Input: part model. Units: mm. Frame: model coordinates. Give positions to 0.01 mm unless a question says otherwise; leave off trailing zeros. Loops run counter-clockwise (first coordinate to the right, second up) from the corner with the lowest first, then second, coordinate; pieces in that order, holes last. Notation, with made-up numbers: (86.25, 77) - (110.25, 77) arc R23 ccw to (110.25, 92) - close; hole circle Ø2 at (-6, 61). An arc over 180 degrees is marked (long way). Answer as a JSON object with one key per item and string values. Group by question number.
(1) Section query B-B (x = -3). Return loops of the section in (y, z), plus the area to 3 significant figures.
(2) Section query A-A (z = 45.5). Return loops of the section in (x, y).
(3) Section query C-C (y = 2.3). Count the separate pieces of the cut face and the enclosed holes in it, plus the area to 3 significant figures.
(4) Material intervals for L1, parallel to X at y = 4.15, z = -12.5; L2, parallel to X at y = 4.6, z = -43; L3, parallel to X at y = 1.4, z = 3, sorted ascending.
Autodesk Inventor part; units mm, degrees
ref_plane "YZ Plane" through (0, 0, 0) normal (1, 0, 0) x (0, 1, 0)
ref_plane "XZ Plane" through (0, 0, 0) normal (0, 1, 0) x (-1, 0, 0)
ref_plane "XY Plane" through (0, 0, 0) normal (0, 0, 1) x (1, 0, 0)
sketch "Sketch1" plane through (0, 0, 0) normal (0, 1, 0) x (-1, 0, 0)
  line L0 (-50.8, 63.5) -> (50.8, 63.5)
  line L1 (50.8, 63.5) -> (50.8, -63.5)
  line L2 (50.8, -63.5) -> (-50.8, -63.5)
  line L3 (-50.8, -63.5) -> (-50.8, 63.5)
  line L4 (-50.8, 63.5) -> (50.8, -63.5) construction
  line L5 (50.8, 63.5) -> (-50.8, -63.5) construction
  point P0 (0, 0)
  point P1 (0, 0)
  dimension "d0" = 101.6
  dimension "d1" = 127
extrude "Plate1" add sketch "Sketch1" along normal blind 5.08
sketch "Sketch2" plane through (0, 5.08, 0) normal (0, 1, 0) x (1, 0, 0)
  line L0 (-50.8, 63.5) -> (50.8, 63.5) construction
  line L1 (0, 63.5) -> (0, -63.5) construction
  line L2 (50.8, -63.5) -> (-50.8, -63.5) construction
  line L3 (-50.8, -63.5) -> (-50.8, 63.5) construction
  point P0 (0, 0)
  point P1 (-37.338, -38.1)
  point P2 (-37.338, -18.542)
  point P3 (37.338, -38.1)
  point P4 (37.338, -18.542)
  dimension "d5" = 19.558
  dimension "d6" = 13.462
  dimension "d18" = 25.4
hole "MotorScrews" at (-37.338, 5.08, 38.1) at (-37.338, 5.08, 18.542) at (37.338, 5.08, 38.1) at (37.338, 5.08, 18.542) direction (0, -1, 0) diameter 3.2766 end through all
sketch "Sketch3" plane through (0, 5.08, 0) normal (0, 1, 0) x (1, 0, 0)
  line L0 (-18.5, -59.9042) -> (18.5, -59.9042)
  line L1 (18.5, -59.9042) -> (18.5, 21.0958)
  line L2 (18.5, 21.0958) -> (-18.5, 21.0958)
  line L3 (-18.5, 21.0958) -> (-18.5, -59.9042)
  line L4 (-18.5, -59.9042) -> (18.5, 21.0958) construction
  line L5 (18.5, -59.9042) -> (-18.5, 21.0958) construction
  point P0 (0, 0)
  point P1 (0, -19.4042)
  point P2 (0, -19.4042)
  dimension "d14" = 37
  dimension "d15" = 81
extrude "BatteryHole" cut sketch "Sketch3" against normal blind 5.08
sketch "Sketch4" plane through (0, 5.08, 0) normal (0, 1, 0) x (1, 0, 0)
  line L0 (18.5, -59.9042) -> (-18.5, -59.9042)
  line L1 (-25.0073, -30.5582) -> (25.0073, -30.5582)
  line L2 (25.0073, -30.5582) -> (25.0073, -24.8469)
  line L3 (25.0073, -24.8469) -> (-25.0073, -24.8469)
  line L4 (-25.0073, -24.8469) -> (-25.0073, -30.5582)
  line L5 (-25.0073, -30.5582) -> (25.0073, -24.8469) construction
  line L6 (25.0073, -30.5582) -> (-25.0073, -24.8469) construction
  point P0 (0, 0)
  point P1 (0, -27.7026)
  point P2 (0, -27.7026)
extrude "MotorWireHoles" cut sketch "Sketch4" against normal blind 5.08
sketch "Sketch5" plane through (0, 5.08, 0) normal (0, 1, 0) x (1, 0, 0)
  line L0 (0, 0) -> (0, 25.4) construction
  line L1 (-50.8, 63.5) -> (50.8, 63.5)
  point P0 (-24.4983, 2.3368)
  point P1 (24.4983, 2.3368)
  point P2 (-24.4983, 60.325)
  point P3 (24.4983, 60.325)
  dimension "d21" = 25.4
  dimension "d22" = 48.9966
  dimension "d23" = 57.9882
  dimension "d24" = 3.175
hole "PiScrews" at (-24.4983, 5.08, -2.3368) at (24.4983, 5.08, -2.3368) at (-24.4983, 5.08, -60.325) at (24.4983, 5.08, -60.325) direction (0, -1, 0) diameter 2.8956 end through all
sketch "Sketch6" plane through (0, 5.08, 0) normal (0, 1, 0) x (1, 0, 0)
  line L0 (-15.4305, 17.2899) -> (-15.4305, 42.6899) construction
  line L1 (-26.2255, 57.1039) -> (-23.0505, 57.1039)
  line L2 (-23.0505, 57.1039) -> (-23.0505, 6.3039)
  line L3 (-23.0505, 6.3039) -> (-26.2255, 6.3039)
  line L4 (-26.2255, 6.3039) -> (-26.2255, 57.1039)
  circle A0 centre (-24.4983, 60.325) radius 1.4478
  line L5 (-4.6355, 57.1039) -> (-7.8105, 57.1039)
  line L6 (-7.8105, 57.1039) -> (-7.8105, 23.8538)
  line L7 (-7.8105, 23.8538) -> (-4.6355, 23.8538)
  line L8 (-4.6355, 23.8538) -> (-4.6355, 57.1039)
  dimension "d33" = 3.175
  dimension "d34" = 50.8
  dimension "d37" = 15.24
extrude "WireHoles" cut sketch "Sketch6" against normal blind 5.08 contours L1 L2 L3 L4 | L8 L7 L6 L5
sketch "Sketch7" plane through (0, 5.08, 0) normal (0, 1, 0) x (1, 0, 0)
  line L0 (-36.0117, 4.0418) -> (-33.4717, 4.0418)
  line L1 (-33.4717, 4.0418) -> (-33.4717, 0.2318)
  line L2 (-33.4717, 0.2318) -> (-36.0117, 0.2318)
  line L3 (-36.0117, 0.2318) -> (-36.0117, 4.0418)
  line L4 (-30.3328, 4.1075) -> (-27.7928, 4.1075)
  line L5 (-27.7928, 4.1075) -> (-27.7928, 0.2975)
  line L6 (-27.7928, 0.2975) -> (-30.3328, 0.2975)
  line L7 (-30.3328, 0.2975) -> (-30.3328, 4.1075)
  point P0 (0, 0)
  dimension "d38" = 2.54
  dimension "d39" = 3.81
  dimension "d40" = 2.54
  dimension "d41" = 3.81
extrude "ZipTieHolder" cut sketch "Sketch7" against normal blind 5.08
equation "\"d12\" = Thickness"
equation "\"d16\" = Thickness"
equation "\"d19\" = Thickness"
equation "\"d30\" = Thickness"
equation "\"d35\" = Thickness"
equation "\"d42\" = Thickness"
equation "\"d4\" = Thickness"
equation "\"BendRadius\" = Thickness"
equation "\"BendReliefWidth\" = Thickness"
equation "\"BendReliefDepth\" = 0.5 * Thickness"
equation "\"CornerReliefSize\" = 4 * Thickness"
equation "\"MinimumRemnant\" = 2 * Thickness"
equation "\"TransitionRadius\" = BendRadius"
equation "\"JacobiRadiusSize\" = BendRadius"
equation "\"GapSize\" = Thickness"
properties part number "pibot_baseplate_battery" material "Polycarbonate, Clear"
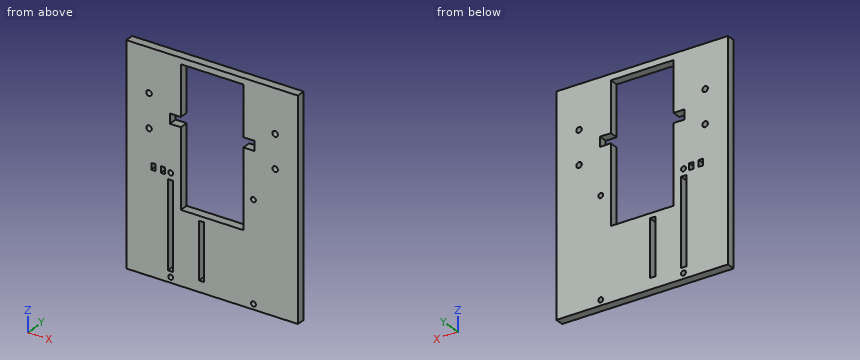
Recorded:
{
 "1": {"outline": "(0, -63.5) - (5.08, -63.5) - (5.08, -21.1) - (0, -21.1) - close; (0, 59.9) - (5.08, 59.9) - (5.08, 63.5) - (0, 63.5) - close", "area": "234 mm^2"},
 "2": {"outline": "(-50.8, 0) - (-18.5, 0) - (-18.5, 5.08) - (-50.8, 5.08) - close; (18.5, 0) - (50.8, 0) - (50.8, 5.08) - (18.5, 5.08) - close"},
 "3": {"separate pieces": "1", "enclosed holes": "13", "area": "9,490 mm^2"},
 "4": {"L1": "x = -50.8 to -26.23, -23.05 to -18.5, 18.5 to 50.8", "L2": "x = -50.8 to -26.23, -23.05 to -7.81, -4.64 to 50.8", "L3": "x = -50.8 to -18.5, 18.5 to 50.8"}
}
